Autodesk Inventor part; units mm, degrees
ref_plane "Work Plane1" through (0, 38.1, -51.05) normal (0, -1, 0) x (1, 0, 0)
ref_plane "Work Plane2" through (0, 0, -25.525) normal (0, 0, 1) x (1, 0, 0)
ref_plane "Work Plane3" through (0, 0, 0) normal (0, -0.7071, -0.7071) x (1, 0, 0)
sketch "Body Sketch" plane through (0, 0, 0) normal (1, 0, 0) x (0, 1, 0)
  line L0 (0, 0) -> (76.2, 0)
  line L1 (76.2, 0) -> (76.2, -51.05)
  line L2 (76.2, -51.05) -> (0, -51.05)
  line L3 (0, -51.05) -> (0, 0)
  dimension "d2" = 76.2
  dimension "d3" = 51.05
extrude "Body Extrude" add sketch "Body Sketch" along normal blind 3
ref_plane "Work Plane1" through (0, 38.1, -51.05) normal (0, -1, 0) x (1, 0, 0)
ref_plane "Work Plane2" through (0, 0, -25.525) normal (0, 0, 1) x (1, 0, 0)
ref_plane "Work Plane3" through (0, 0, 0) normal (0, -0.7071, -0.7071) x (1, 0, 0)
ref_plane "Work Plane4" through (0, 76.2, 0) normal (0, 0.7071, -0.7071) x (-1, 0, 0)
sketch "Hole Sketch" plane through (3, 0, 0) normal (1, 0, 0) x (0, 0, -1)
  line L0 (0, 0) -> (6.35, 0) construction
  line L1 (6.35, 0) -> (6.35, 6.35) construction
  line L2 (6.35, 6.35) -> (0, 6.35) construction
  line L3 (0, 6.35) -> (0, 0) construction
  point P0 (44.45, 6.35)
  point P1 (-19.2059, 16.3555)
  point P2 (6.35, 69.85)
  point P3 (44.45, 69.85)
  dimension "d4" = 6.35
  dimension "d55" = 38.1
  dimension "d56" = 63.5
hole "Hole" at (3, 6.35, -6.35) at (3, 69.85, -6.35) at (3, 69.85, -44.45) at (3, 6.35, -44.45) direction (-1, 0, 0) diameter 4.25 end through all
fillet "Fillet2" radius 5 4 edges at (1.5, 76.2, 0) (1.5, 0, 0) (1.5, 76.2, -51.05) (1.5, 0, -51.05)
equation "\"d54\" = FilletRadius"
equation "\"d4\" = 0.5 * GridSpacing"
equation "\"d5\" = HoleDiam"
equation "\"Thickness\" = 3"
equation "\"GridSpacing\" = 12.7"
equation "\"HoleDiam\" = 4.25"
equation "\"FilletRadius\" = 5"
properties part number "Rotary Actuator Platform Design 2" material "Acetal Resin, Black"
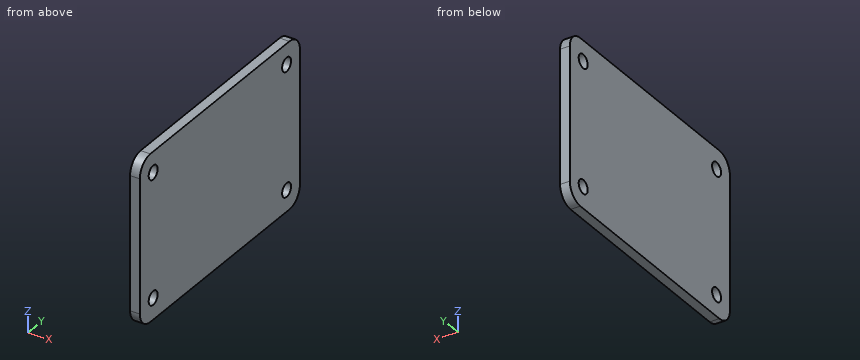
CAD build for the part. Positions are in the model's coordinates, mm. Coordinates: 2 decimals unless noted, no trailing zeros. Order: outer loops, then holes, each group sorted by start corner. A loop starts at its lowest first (then second) coordinate and runs counter-clockwise, first axis right, second up.
(1) Drill centre lines: L1, parallel to Z at x = 1.3, y = 6.35 (3 decimals); L2, parallel to Y at x = 0.65, z = -44.45 (3 decimals); L3, parallel to Y at x = 0.55, z = -6. Where is each one in solid material? Low to high.
Solution:
L1: z = -51.05 to -46.575, -42.325 to -8.475, -4.225 to 0
L2: y = 0 to 4.225, 8.475 to 67.725, 71.975 to 76.2
L3: y = 0 to 4.25, 8.45 to 67.75, 71.95 to 76.2
(2) Saw through at A-A, the plane y = 6.35. Write the cut outline in (x, z) (3 decimals).
Solution:
outline: (0, -51.05) - (3, -51.05) - (3, -46.575) - (0, -46.575) - close; (0, -42.325) - (3, -42.325) - (3, -8.475) - (0, -8.475) - close; (0, -4.225) - (3, -4.225) - (3, 0) - (0, 0) - close
(3) Saw through at B-B, the plane x = 2.3. Write the cut outline in (y, z) (3 decimals), and give its area (3 significant figures).
Solution:
outline: (0, -46.05) arc R5 ccw to (5, -51.05) - (71.2, -51.05) arc R5 ccw to (76.2, -46.05) - (76.2, -5) arc R5 ccw to (71.2, 0) - (5, 0) arc R5 ccw to (0, -5) - close; hole circle Ø4.25 at (6.35, -44.45); hole circle Ø4.25 at (6.35, -6.35); hole circle Ø4.25 at (69.85, -44.45); hole circle Ø4.25 at (69.85, -6.35)
area: 3,810 mm2
(4) Pin check, flat tip, straight feed: pin 1 Ø5 at (y, z) = (6.35, -44.45) entering from -X. Stop position of the tip, or through.
Solution:
pin 1: stops at x = 0
(5) Saw through at C-C, the plane z = -6.35. Write the cut outline in (x, y) (3 decimals), and give its area (3 significant figures).
Solution:
outline: (0, 0) - (3, 0) - (3, 4.225) - (0, 4.225) - close; (0, 8.475) - (3, 8.475) - (3, 67.725) - (0, 67.725) - close; (0, 71.975) - (3, 71.975) - (3, 76.2) - (0, 76.2) - close
area: 203 mm2
